Work out the finished part from the listing and answer in its coordinate system (mm). A direction names the side the tool comes from. Give positions to 0.01 mm unless a question says otherwise; leave off trailing zeros. Loops run counter-clockwise (first coordinate to the right, second up) from the corner with the lowest first, then second, coordinate; pieces in that order, holes last.
```python
from build123d import *

# Parameters (mm, degrees)
F0_W     = 101.6
F0_H     = 6.35
F2_R     = 6.35
F3_DEPTH = 12.446


with BuildPart() as f1:
    # F0 (on Front) → F1 (revolve)
    with BuildSketch(Plane.XZ):
        with Locations((-9.9456323085, 41.275)):
            Rectangle(F0_W, F0_H)
    revolve(axis=Axis((-36.8506624945, 0, 0), (1, 0, 0)))

    # F2 (on Right) → F3 (join)
    with BuildSketch(Plane.YZ):
        with BuildLine():
            ThreePointArc((-7.5566940289, 20.9008851572), (0, 22.225), (7.5566940289, 20.9008851572))
            add(Edge.make_bspline(
                [(7.5566940289, 20.9008851572), (8.1307940533, 23.1498468847), (9.2859974924, 27.6739638996), (15.6936893767, 31.1495582912), (17.4205445494, 32.8370367229), (18.1234413691, 33.5134431675)],
                knots=[0, 0, 0, 0, 0.3703034477, 0.7423878019, 1, 1, 1, 1], degree=3))
            ThreePointArc((18.1234413691, 33.5134431675), (0, 38.1), (-18.1234413691, 33.5134431675))
            add(Edge.make_bspline(
                [(-7.5566940289, 20.9008851572), (-8.1307940533, 23.1498468847), (-9.2859974924, 27.6739638996), (-15.6936893767, 31.1495582912), (-17.4205445494, 32.8370367229), (-18.1234413691, 33.5134431675)],
                knots=[0, 0, 0, 0, 0.3703034477, 0.7423878019, 1, 1, 1, 1], degree=3))
        make_face()
        with BuildLine():
            ThreePointArc((7.5566940289, -20.9008851572), (18.1920057964, -12.7672060414), (22.225, 0))
            ThreePointArc((22.225, 0), (18.1920057964, 12.7672060414), (7.5566940289, 20.9008851572))
            ThreePointArc((7.5566940289, 20.9008851572), (0, 22.225), (-7.5566940289, 20.9008851572))
            ThreePointArc((-7.5566940289, 20.9008851572), (-22.225, 0), (-7.5566940289, -20.9008851572))
            ThreePointArc((-7.5566940289, -20.9008851572), (0, -22.225), (7.5566940289, -20.9008851572))
        make_face()
        Circle(F2_R, mode=Mode.SUBTRACT)
        with BuildLine():
            add(Edge.make_bspline(
                [(7.5566940289, -20.9008851572), (8.1307940533, -23.1498468847), (9.2859974924, -27.6739638996), (15.6936893767, -31.1495582912), (17.4205445494, -32.8370367229), (18.1234413691, -33.5134431675)],
                knots=[0, 0, 0, 0, 0.3703034477, 0.7423878019, 1, 1, 1, 1], degree=3))
            ThreePointArc((7.5566940289, -20.9008851572), (0, -22.225), (-7.5566940289, -20.9008851572))
            add(Edge.make_bspline(
                [(-7.5566940289, -20.9008851572), (-8.1307940533, -23.1498468847), (-9.2859974924, -27.6739638996), (-15.6936893767, -31.1495582912), (-17.4205445494, -32.8370367229), (-18.1234413691, -33.5134431675)],
                knots=[0, 0, 0, 0, 0.3703034477, 0.7423878019, 1, 1, 1, 1], degree=3))
            ThreePointArc((-18.1234413691, -33.5134431675), (0, -38.1), (18.1234413691, -33.5134431675))
        make_face()
    extrude(amount=-F3_DEPTH)


solid = f1.part
```
Q1. Section C-C on x = -8.5 is taken. State how many separate pieces and enclosed holes the cut face has, plus the area to 3 significant figures.
Q2. Determine the mould class of faces 1 (the face through (40.854, -20, -33)), 2 (the face through (-9.23, -37.48, 23.9)), 3 (the face through (0, 0, -8)), 4 (the face through (-9.234, 23.183, -30.235)) for opening direction Y: +Y half, -Y half, draft (parallel to the pull), parting line (faces both ways), or undercut.
Q3. Given pin 1 (1 mm diameter, centred on x = -17.5, y = -5.5, fed in from +Z); pin 2 (6 mm diameter, centred on x = 30, z = -6, fed in from +Y); pin 3 (6 mm diameter, centred on y = -15.5, z = 6, fed in from +X), each flat-ended and moving along its own axis, determine where each tip first touches the part or whether it passes through.
Q4. Which of the six approach directions +Z, -Z, +X, -X, +Y, -Y give full straight-line access (tool end or side, diameter ignored) to faces 5 (the face through (-60.746, -20, -33)), 6 (the face through (-6.14, -22.22, 0.38)), 7 (the face through (-12.446, 0, -8))?
Q5. Section A-A on y = 0 is taken. Give the vertices of the cut face in (x, z), plus the area to 3 significant figures.
Q6. Consider line 1 along Z through (x, y) = (-10, 0); line 2 along Z through (x, y) = (9, -1); line 3 along Y through (x, z) = (-3.5, 10.5). Determine where each line is inside the solid, lowest interval first.
Q7. Section B-B on x = 19 is taken. Give the vertices of the cut face in (y, z), plus the area to 3 significant figures.
Q8. Section D-D on y = 29 is taken. Give the vertices of the cut face in (x, z).
Check result:
1. separate pieces: 1
1. enclosed holes: 3
1. area: 3,840 mm2
2. face 1: draft
2. face 2: parting line
2. face 3: undercut
2. face 4: undercut
3. pin 1: stops at z = 44.17
3. pin 2: stops at y = 44.35
3. pin 3: stops at x = 0
4. face 5: +Z, -Z, -X, +Y, -Y
4. face 6: +X, -X
4. face 7: -X
5. outline: (-60.75, -44.45) - (40.85, -44.45) - (40.85, -38.1) - (0, -38.1) - (0, -6.35) - (-12.45, -6.35) - (-12.45, -38.1) - (-60.75, -38.1) - close; (-60.75, 38.1) - (-12.45, 38.1) - (-12.45, 6.35) - (0, 6.35) - (0, 38.1) - (40.85, 38.1) - (40.85, 44.45) - (-60.75, 44.45) - close
5. area: 2,080 mm2
6. line 1: z = -44.45 to -6.35, 6.35 to 44.45
6. line 2: z = -44.44 to -38.09, 38.09 to 44.44
6. line 3: y = -43.19 to -36.62, -19.59 to 19.59, 36.62 to 43.19
7. outline: circle Ø88.9 at (0, 0); hole circle Ø76.2 at (0, 0)
7. area: 1,650 mm2
8. outline: (-60.75, -33.69) - (40.85, -33.69) - (40.85, -24.71) - (-60.75, -24.71) - close; (-60.75, 24.71) - (40.85, 24.71) - (40.85, 33.69) - (-60.75, 33.69) - close
